For this review, take the finished solid that the model builds, in its own axes (mm). Face numbers are marked on the shaded views. A direction names the side the tool comes from. Round coordinates to 2 decimals unless told otherwise and drop trailing zeros. Write each loop counter-clockwise with the first axis right and the second up, starting at its lowest first coordinate (ties: lowest second). Pieces come first, ordered by that corner, then holes. Notation, with made-up numbers: M 65.5,23.25 L 99.5,23.25 A33 cw 99.5,51.25 Z; hole C -3,2.5 d4. An arc over 180 degrees is marked long. Write each question's results on one line, items separated by ' | '. Start each with the question number.
```python
from build123d import *

# Parameters (mm, degrees)
BOSS_EXTRUDE1_DEPTH = 22.5
SKETCH2_R           = 16.25
CUT_EXTRUDE1_DEPTH  = 10
SKETCH3_R           = 7
CUT_EXTRUDE2_DEPTH  = 25


with BuildPart() as part:
    # Sketch1 → Boss-Extrude1 (new body, symmetric)
    with BuildSketch(Plane.XY):
        Polygon((-17.5, 30.310889132), (17.5, 30.310889132), (35, 0), (17.5, -30.310889132), (-17.5, -30.310889132), (-35, 0), align=None)
    extrude(amount=BOSS_EXTRUDE1_DEPTH, both=True)

    # Sketch2 → Cut-Extrude1 (cut)
    with BuildSketch(Plane.XY.offset(22.5)):
        Circle(SKETCH2_R)
    cut_extrude1 = extrude(amount=-CUT_EXTRUDE1_DEPTH, mode=Mode.SUBTRACT)

    # Mirror1: Cut-Extrude1 across plane
    add(cut_extrude1.mirror(Plane.XY), mode=Mode.SUBTRACT)

    # Sketch3 → Cut-Extrude2 (cut)
    with BuildSketch(Plane(origin=(0, 0, -12.5), x_dir=(-1, 0, 0), z_dir=(0, 0, -1))):
        Circle(SKETCH3_R)
    extrude(amount=-CUT_EXTRUDE2_DEPTH, mode=Mode.SUBTRACT)


solid = part.part
```
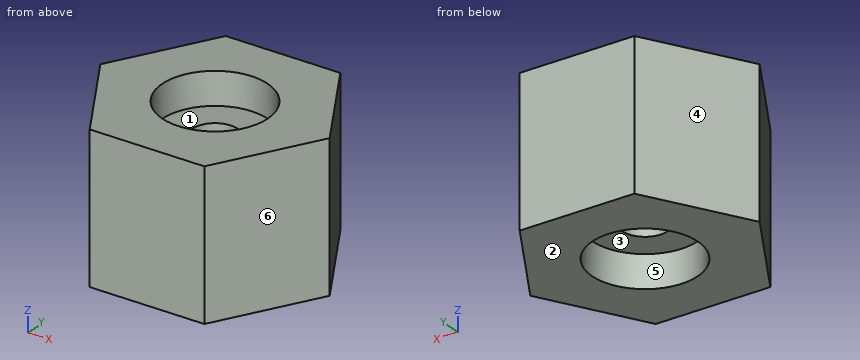
Item 1: For the marked faces 1, 2 and 3, list the 3-axis set-ups (+Z, -Z, +X, -X, +Y, -Y) from which the entire face can be reached by the end or side of a thin tool; tool diameter is ignored.
Item 2: We need section C-C on z = 18. State the section outline as (x, y) points.
Item 3: Insertion check: P1, Ø2, axis at x = -19.5, z = 13.5, coming from the +Y side; P2, Ø10, axis at x = 5, y = -6, coming from the -Z side; P3, Ø2, axis at x = -13.5, y = -4.5, coming from the +Z side; P4, Ø8.5, axis at x = 0, y = 0, coming from the -Z side. Each pin has a flat end and moves straight along its axis. Give the tip position at first contact, or say it passes through.
Item 4: We need section D-D on y = -9.5. State the section outline as (x, z) points, then the cut area to 3 significant figures.
Item 5: Mouldability with a two-part tool opening along Y and no side actions: class the marked faces 4, 5 and 6 as pulls with the +Y half, pulls with the -Y half, needs draft (parallel to the pull), parting line crosses it, or undercut.
Item 6: We need section A-A on x = 0. State the section outline as (y, z) points.
Item 7: We need section B-B on z = 9.5. State the section outline as (x, y) points, then the cut area to 3 significant figures.
Item 8: For probe 1 along Y at (x, z) = (0, -4.75); probe 2 along Y at (x, z) = (0, 19.75); probe 3 along X at (y, z) = (6.5, 17.5), list the stretches that pass through material, from the lowest coordinate up.
Numbers:
1) face 1: +Z | face 2: -Z, +X, -X, +Y, -Y | face 3: -Z
2) outline: M -35,0 L -17.5,-30.31 L 17.5,-30.31 L 35,0 L 17.5,30.31 L -17.5,30.31 Z; hole C 0,0 d32.5
3) P1: stops at y = 28.58 | P2: stops at z = -12.5 | P3: stops at z = 12.5 | P4: passes through
4) outline: M -29.52,-22.5 L -13.18,-22.5 L -13.18,-12.5 L 13.18,-12.5 L 13.18,-22.5 L 29.52,-22.5 L 29.52,22.5 L 13.18,22.5 L 13.18,12.5 L -13.18,12.5 L -13.18,22.5 L -29.52,22.5 Z | area: 2,130 mm^2
5) face 4: pulls with the +Y half | face 5: undercut | face 6: pulls with the -Y half
6) outline: M -30.31,-22.5 L -16.25,-22.5 L -16.25,-12.5 L -7,-12.5 L -7,12.5 L -16.25,12.5 L -16.25,22.5 L -30.31,22.5 Z; M 7,-12.5 L 16.25,-12.5 L 16.25,-22.5 L 30.31,-22.5 L 30.31,22.5 L 16.25,22.5 L 16.25,12.5 L 7,12.5 Z
7) outline: M -35,0 L -17.5,-30.31 L 17.5,-30.31 L 35,0 L 17.5,30.31 L -17.5,30.31 Z; hole C 0,0 d14 | area: 3,030 mm^2
8) probe 1: y = -30.31 to -7, 7 to 30.31 | probe 2: y = -30.31 to -16.25, 16.25 to 30.31 | probe 3: x = -31.25 to -14.89, 14.89 to 31.25
